For this review, take the finished solid that the model builds, in its own axes (mm). Give positions to 0.01 mm unless a question says otherwise; leave off trailing zeros. Order: outer loops, then holes, each group sorted by start corner. A loop starts at its lowest first (then second) coordinate and runs counter-clockwise, first axis right, second up. Notation, with made-up numbers: (-18, -37.75) -> (40, -37.75) arc R8 ccw to (40, -24.75) -> close; hole circle Ø3 at (73, 18). An arc over 180 degrees is marked (long way). One line per item, written item: value. Start each with the question number.
from build123d import *

# Parameters (mm, degrees)
SKETCH1_R           = 82.5
BOSS_EXTRUDE1_DEPTH = 152.4
SKETCH3_W           = 217.5
SKETCH3_H           = 152.307162038
BOSS_EXTRUDE2_DEPTH = 1.5
CIRPATTERN1_COUNT   = 3


with BuildPart() as part:
    # Sketch1 → Boss-Extrude1 (new body)
    with BuildSketch(Plane(origin=(0, 0, 0), x_dir=(1, 0, 0), z_dir=(0, 1, 0))):
        with Locations(Location((0, 0, 0), (0, 0, 90))):
            Circle(SKETCH1_R)
    extrude(amount=BOSS_EXTRUDE1_DEPTH)

    # Sketch3 → Boss-Extrude2 (add, symmetric)
    with BuildSketch(Plane(origin=(-2.65772165, 0.092809685, 0), x_dir=(0, 0, -1), z_dir=(0.9993908270190958, -0.03489949670250104, 0))):
        with Locations((-108.75, 76.153581019)):
            Rectangle(SKETCH3_W, SKETCH3_H)
    boss_extrude2 = extrude(amount=BOSS_EXTRUDE2_DEPTH, both=True)

    # CirPattern1: Boss-Extrude2 ×3 about axis
    cirpattern1_axis = Axis((0, 0, 0), (0, 1, 0))
    for i in range(1, CIRPATTERN1_COUNT):
        add(boss_extrude2.rotate(cirpattern1_axis, i * 360 / CIRPATTERN1_COUNT))


solid = part.part
Q1. Mouldability with a two-part tool opening along X and no side actions: class faces 1 (the flat face through (-1, 152.4, 1)), 2 (the cylindrical face through (80.54, 75.13, 17.88)) as pulls with the +X half, pulls with the -X half, needs draft (parallel to the pull), parting line crosses it, or undercut.
Q2. For pin 1 Ø1.5 at (x, y) = (95, 43) entering from +Z; pin 2 Ø8 at (x, y) = (-32, 81.5) entering from +Z; pin 3 Ø8 at (x, y) = (-36, 39.5) entering from -Z; pin 4 Ø3 at (x, z) = (-20, -60.5) entering from -Y, all flat-tipped, find the tip position at first contact; note any pin that passes through.
Q3. For line 1 along X through (y, z) = (91, -69); line 2 along X through (y, z) = (61.5, -49); line 3 along X through (y, z) = (45, 0), list the stretches that pass through material, from the lowest coordinate up.
Q4. Take a section at D-D (z = 0). State the section outline as (x, y) points.
Q5. Take a section at B-B (y = 94.5). State the section outline as (x, z) points, and give its area (3 significant figures).
Q6. Take a section at A-A (z = -65.5). State the section outline as (x, y) points.
Q7. Take a section at C-C (x = -119.5). State the section outline as (y, z) points.
Answers below:
1. face 1: needs draft
1. face 2: undercut
2. pin 1: stops at z = -51.34
2. pin 2: stops at z = 77.6
2. pin 3: stops at z = -76.04
2. pin 4: stops at y = 0
3. line 1: x = -123.55 to -117.54, -45.22 to 45.22, 115.48 to 121.48
3. line 2: x = -86.85 to -80.84, -66.37 to 66.37, 82.9 to 88.9
3. line 3: x = -82.5 to 82.5
4. outline: (-82.5, 0) -> (82.5, 0) -> (82.5, 152.4) -> (-82.5, 152.4) -> close
5. outline: (-189.43, -106.9) -> (-187.93, -109.5) -> (-71.01, -41.99) arc R82.5 ccw to (70.35, -43.09) -> (187.29, -110.6) -> (188.79, -108) -> (71.87, -40.5) arc R82.5 ccw to (2.14, 82.47) -> (2.14, 217.5) -> (-0.86, 217.5) -> (-0.86, 82.5) arc R82.5 ccw to (-72.49, -39.38) -> close
5. area: 22,600 mm²
6. outline: (-121.76, 152.25) -> (-111.13, 0.04) -> (-105.14, 0.15) -> (-115.77, 152.36) -> close; (-50.16, 0) -> (50.16, 0) -> (50.16, 152.4) -> (-50.16, 152.4) -> close; (105.14, 152.25) -> (115.77, 0.04) -> (121.76, 0.15) -> (111.13, 152.36) -> close
7. outline: (0.04, -70.33) -> (0.15, -73.79) -> (152.36, -67.66) -> (152.25, -64.19) -> close
